Autodesk Inventor part; units mm, degrees
ref_plane "Work Plane1" through (-232.5644, -49.9301, 5) normal (0, -1, 0) x (1, 0, 0)
ref_plane "YZ Plane" through (0, 0, 0) normal (1, 0, 0) x (0, 1, 0)
ref_plane "XZ Plane" through (0, 0, 0) normal (0, 1, 0) x (-1, 0, 0)
sketch "Sketch1" plane through (0, 0, 0) normal (0, 0, 1) x (1, 0, 0)
  circle A0 centre (0, 0) radius 17.5
  dimension "d0" = 35
extrude "Extrusion1" add sketch "Sketch1" along normal blind 5
sketch "Sketch2" plane through (0, 0, 5) normal (0, 0, 1) x (1, 0, 0)
  line L0 (25, 1.5) -> (-25, 1.5)
  line L1 (-25, 1.5) -> (-25, -1.5)
  line L2 (-25, -1.5) -> (25, -1.5)
  line L3 (25, -1.5) -> (25, 1.5)
  line L4 (25, 1.5) -> (-25, -1.5) construction
  line L5 (-25, 1.5) -> (25, -1.5) construction
  arc A0 (-8.8619, 3.6913) -> (8.9371, 3.5055) centre (0, 0) ccw
  circle A1 centre (0, 0) radius 17.5
  circle A2 centre (0, 0) radius 17.5
  line L6 (17.4356, -1.5) -> (-22.5, -1.5)
  line L7 (-22.5, -1.5) -> (-22.5, -6.5)
  line L8 (-22.5, -6.5) -> (17.4356, -6.5)
  line L9 (17.4356, -6.5) -> (17.4356, -1.5)
  line L10 (17.4356, 1.5) -> (-22.5, 1.5)
  line L11 (-22.5, 1.5) -> (-22.5, 6.5)
  line L12 (-22.5, 6.5) -> (17.4356, 6.5)
  line L13 (17.4356, 6.5) -> (17.4356, 1.5)
  point P0 (-3.75, -16.4)
  point P1 (16.2481, 6.5)
  point P2 (-16.2481, 6.5)
  point P3 (-17.4356, 1.5)
  point P4 (17.4356, 1.5)
  point P5 (16.2481, -6.5)
  point P6 (17.4356, -1.5)
  point P7 (-17.4356, -1.5)
  point P8 (-16.2481, -6.5)
  dimension "d3" = 50
  dimension "d4" = 3
  dimension "d5" = 5
  dimension "d6" = 5
extrude "Extrusion2" add sketch "Sketch2" along normal blind 50 contours L0 A1 L12 | A1 L8 A0 L2 | A0 L8 L2 | A0 L8 A1 L2
sketch "Sketch3" plane through (-16.2481, 6.5, 5) normal (0, 1, 0) x (1, 0, 0)
  line L0 (0, 0) -> (32.4962, 0)
  line L1 (0, 0) -> (0, -50)
  line L2 (32.4962, -50) -> (0, -50)
  line L3 (32.4962, 0) -> (32.4962, -50)
  line L4 (0, 0) -> (0, -50)
  line L5 (32.4962, 0) -> (32.4962, -50)
  line L6 (0, 0) -> (32.4962, -50)
  line L7 (32.4962, -50) -> (0, -50)
  line L8 (0, -50) -> (32.4962, 0)
  line L9 (27.6217, -7.5) -> (4.8744, -7.5)
  line L10 (4.8744, -7.5) -> (4.8744, -42.5)
  line L11 (4.8744, -42.5) -> (27.6217, -42.5)
  line L12 (27.6217, -42.5) -> (27.6217, -7.5)
  line L13 (27.6217, -7.5) -> (4.8744, -42.5) construction
  line L14 (4.8744, -7.5) -> (27.6217, -42.5) construction
  circle A0 centre (27.6217, -42.5) radius 1.5
  circle A1 centre (4.8744, -42.5) radius 1.5
  circle A2 centre (4.8744, -7.5) radius 1.5
  circle A3 centre (27.6217, -7.5) radius 1.5
  point P0 (16.2481, 5)
  point P1 (16.2481, -25)
  dimension "d9" = 35
  dimension "d10" = 3
  dimension "d11" = 3
  dimension "d12" = 3
  dimension "d13" = 3
extrude "Extrusion3" cut sketch "Sketch3" against normal through all contours A2 L9 L6 | L6 L10 A2 | A3 L12 L8 | L8 L9 A3 | A1 L10 L8 | L8 L11 A1 | L9 A2 L6 | L6 A2 L10 | A0 L11 L6 | L6 L12 A0 | L12 A3 L8 | L8 A3 L9 | L10 A1 L8 | L8 A1 L11 | L11 A0 L6 | L6 A0 L12
sketch "Sketch4" plane through (-16.2481, -6.5, 5) normal (0, -1, 0) x (1, 0, 0)
  line L0 (13.75, 50) -> (18.75, 50)
  line L1 (18.75, 50) -> (18.75, 0)
  line L2 (18.75, 0) -> (13.75, 0)
  line L3 (13.75, 0) -> (13.75, 50)
  line L4 (0, 50) -> (32.4962, 50)
  line L5 (32.4962, 0) -> (0, 0)
  line L6 (0, 0) -> (0, 50)
  point P0 (16.2481, -5)
  dimension "d16" = 0
  dimension "d17" = 0
  dimension "d18" = 5
  dimension "d19" = 13.75
ref_plane "Work Plane1" through (-232.5644, -49.9301, 5) normal (0, -1, 0) x (1, 0, 0)
extrude "Extrusion4" add sketch "Sketch4" along normal up to surface (43.4301 mm away) contours L0 L1 L2 L3
sketch "Sketch5" plane through (-2.4981, -6.5, 5) normal (-1, 0, 0) x (0, 0, 1)
  ellipse E0 centre (25.0308, -20) end of major axis (25.0308, -23.5) minor radius 3.5
  point P0 (-5, 6.5)
extrude "Extrusion5" cut sketch "Sketch5" against normal through all
sketch "Sketch6" plane through (-2.4981, -6.5, 5) normal (-1, 0, 0) x (0, 0, 1)
  circle A0 centre (25.0308, -31.22) radius 2.08
  point P0 (-5, 6.5)
extrude "Extrusion6" cut sketch "Sketch6" against normal up to surface (5 mm away)
sketch "Sketch7" plane through (-2.4981, -6.5, 5) normal (-1, 0, 0) x (0, 0, 1)
  circle A0 centre (33.7808, -40.11) radius 1.5
  circle A1 centre (16.2808, -40.11) radius 1.5
  point P0 (-5, 6.5)
extrude "Extrusion7" cut sketch "Sketch7" against normal blind 50
sketch "Sketch8" plane through (-2.4981, -49.9301, 5) normal (0, -1, 0) x (1, 0, 0)
  line L0 (0, 0) -> (0, 50)
  line L1 (5, 0) -> (0, 0)
  line L2 (5, 50) -> (5, 0)
  line L3 (0, 50) -> (5, 50)
  point P0 (2.4981, -5)
extrude "Extrusion8" add sketch "Sketch8" along normal blind 10
properties part number "arm - servo mount" material "PET Plastic"
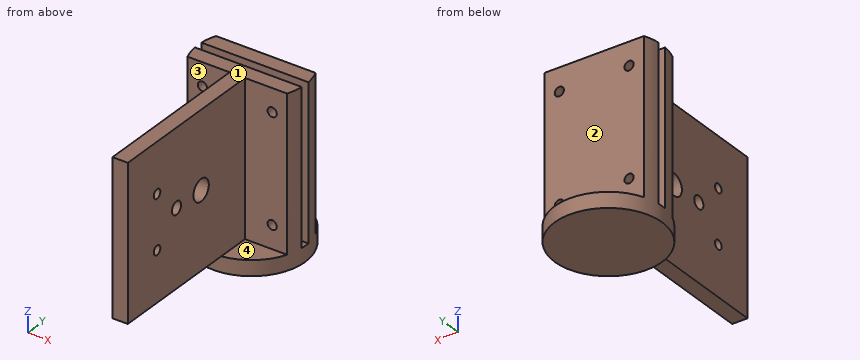
Source: CAD feature listing. Evaluate the final solid. Frame: model axes, mm. Face numbers are marked on the shaded views. A direction names the side the tool comes from. Round coordinates to 2 decimals unless told otherwise and drop trailing zeros. Loops run counter-clockwise (first coordinate to the right, second up) from the corner with the lowest first, then second, coordinate; pieces in that order, holes last. Notation, with made-up numbers: M -5,38.25 L 34,38.25 A9 ccw 34,50.25 Z; hole C 60.25,18.25 d4. An arc over 180 degrees is marked long. Use a Markdown table: item, result. Add a question column.
1. Ray query, line 1 along Y through (x, z) = (-1.5, 39); line 2 along Y through (x, z) = (-11, 8); line 3 along Z through (x, y) = (0, -46). Return the intervals inside material, ascending. Write a range as [from, to].
2. Set-up query: the marked faces 1, 2, 3 and 4. Return all of +Z, -Z, +X, -X, +Y, -Y with unobstructed straight access to the full face (end or side cutting, diameter ignored); none if empty.
3. Cut plane B-B, the plane y = -46.61. Output: boundary loops of the cut face in (x, z).
4. Cut plane C-C, the plane z = 12.5. Output: boundary loops of the cut face in (x, y).
5. Cut plane A-A, the plane z = 6. Output: boundary loops of the cut face in (x, y).
6. Cut plane D-D, the plane y = -37.72. Output: boundary loops of the cut face in (x, z), and give its area (3 significant figures).
7. Contact query for flat-ended pins moving along their axis: pin 1 (3.5 mm diameter, centred on x = 11.37, z = 47.5, fed in from +Y); pin 2 (3 mm diameter, centred on x = 8.5, y = -9.5, fed in from +Z); pin 3 (10 mm diameter, centred on y = -33, z = 28.5, fed in from +X). Output: stop coordinate, or through.
Solution:
| question | item | result |
|---|---|---|
| 1 | line 1 | y = [-59.93, -48.09], [-45.13, -1.5], [1.5, 6.5] |
| 1 | line 2 | y = [-6.5, -1.5], [1.5, 6.5] |
| 1 | line 3 | z = [5, 19.91], [22.65, 37.41], [40.15, 55] |
| 2 | face 1 | +Z, +X, -X, +Y, -Y |
| 2 | face 2 | +Z, +X, -X, +Y |
| 2 | face 3 | +Z, -X, -Y |
| 2 | face 4 | +Z, +X, -Y |
| 3 | outline | M -2.5,5 L 2.5,5 L 2.5,19.78 L -2.5,19.78 Z; M -2.5,22.78 L 2.5,22.78 L 2.5,37.28 L -2.5,37.28 Z; M -2.5,40.28 L 2.5,40.28 L 2.5,55 L -2.5,55 Z |
| 4 | outline | M -17.44,-1.5 A17.5 ccw -16.25,-6.5 L -12.87,-6.5 L -12.87,-1.5 Z; M -17.44,1.5 L -12.87,1.5 L -12.87,6.5 L -16.25,6.5 A17.5 ccw Z; M -9.87,-6.5 L -2.5,-6.5 L -2.5,-59.93 L 2.5,-59.93 L 2.5,-6.5 L 9.87,-6.5 L 9.87,-1.5 L -9.87,-1.5 Z; M -9.87,1.5 L 9.87,1.5 L 9.87,6.5 L -9.87,6.5 Z; M 12.87,-6.5 L 16.25,-6.5 A17.5 ccw 17.44,-1.5 L 12.87,-1.5 Z; M 12.87,1.5 L 17.44,1.5 A17.5 ccw 16.25,6.5 L 12.87,6.5 Z |
| 5 | outline | M -17.44,-1.5 A17.5 ccw -16.25,-6.5 L -2.5,-6.5 L -2.5,-59.93 L 2.5,-59.93 L 2.5,-6.5 L 16.25,-6.5 A17.5 ccw 17.44,-1.5 Z; M -17.44,1.5 L 17.44,1.5 A17.5 ccw 16.25,6.5 L -16.25,6.5 A17.5 ccw Z |
| 6 | outline | M -2.5,5 L 2.5,5 L 2.5,27.95 L -2.5,27.95 Z; M -2.5,32.11 L 2.5,32.11 L 2.5,55 L -2.5,55 Z |
| 6 | area | 229 mm2 |
| 7 | pin 1 | stops at y = 6.5 |
| 7 | pin 2 | stops at z = 5 |
| 7 | pin 3 | stops at x = 2.5 |
